from build123d import *

# Parameters (mm, degrees)
F0_R     = 7.14375
F0_R_2   = 33.3375
F0_R_3   = 8.509
F0_R_4   = 8.89
F0_R_5   = 137.31875
F1_DEPTH = 4.7625


with BuildPart() as f1:
    # F0 (on Right) → F1 (new body)
    with BuildSketch(Plane.YZ):
        with BuildLine():
            Line((-271.696104, -5.952033), (-271.696104, -221.890895))
            ThreePointArc((-271.696104, -221.890895), (-257.051472, -257.246163), (-221.696204, -271.890795))
            Line((-221.696204, -271.890795), (-6.535242, -271.890795))
            Line((-6.535242, -271.890795), (254.987282, -10.17713))
            ThreePointArc((254.987282, -10.17713), (250.021545, 250.150476), (-10.30357, 255.245143))
            Line((-10.30357, 255.245143), (-271.696104, -5.952033))
        make_face()
        with Locations((-244.518688, -244.572155)):
            Circle(F0_R, mode=Mode.SUBTRACT)
        with Locations((-34.20458, -244.572155)):
            Circle(F0_R, mode=Mode.SUBTRACT)
        with Locations((-244.518688, -34.39127)):
            Circle(F0_R, mode=Mode.SUBTRACT)
        with Locations((-190.572923, -34.39127)):
            Circle(F0_R, mode=Mode.SUBTRACT)
        with Locations((-127.660375, -34.39127)):
            Circle(F0_R_2, mode=Mode.SUBTRACT)
        with Locations((-64.7478, -34.39127)):
            Circle(F0_R, mode=Mode.SUBTRACT)
        with Locations((2.731567, 2.773934)):
            Circle(F0_R_3, mode=Mode.SUBTRACT)
        with Locations((81.847131, -140.540435)):
            Circle(F0_R, mode=Mode.SUBTRACT)
        with Locations((117.685388, -44.901637)):
            Circle(F0_R_3, mode=Mode.SUBTRACT)
        with Locations((231.706395, 2.789326)):
            Circle(F0_R_3, mode=Mode.SUBTRACT)
        with Locations((-140.560552, 81.726329)):
            Circle(F0_R, mode=Mode.SUBTRACT)
        with Locations((-44.795135, 117.578861)):
            Circle(F0_R_3, mode=Mode.SUBTRACT)
        with Locations((2.655392, 231.961842)):
            Circle(F0_R_4, mode=Mode.SUBTRACT)
        with Locations((117.211272, 117.405963)):
            Circle(F0_R_5, mode=Mode.SUBTRACT)
        with Locations((279.937693, 117.578861)):
            Circle(F0_R_3, mode=Mode.SUBTRACT)
        with Locations((117.600933, 279.905917)):
            Circle(F0_R_3, mode=Mode.SUBTRACT)
        with Locations((231.809138, 231.996234)):
            Circle(F0_R_3, mode=Mode.SUBTRACT)
    extrude(amount=F1_DEPTH)


solid = f1.part
Design review of the part built by this model. Coordinates are the model's own, in mm. Round coordinates to 2 decimals unless told otherwise and drop trailing zeros. Loops run counter-clockwise (first coordinate to the right, second up) from the corner with the lowest first, then second, coordinate; pieces in that order, holes last. Notation, with made-up numbers: (13, 54.5) - (20, 54.5) arc R32 cw to (20, 91.5) - close; hole circle Ø5 at (-25.5, 45). An arc over 180 degrees is marked (long way). One line per item, written item: value. Start each with the question number.
1) To check wall thickness, follow L1, parallel to Y at x = 2.65, z = -246.5; L2, parallel to Y at x = 3.25, z = 7; L3, parallel to Y at x = 1.95, z = 58. State the ranges of each line that lie inside material, in increasing order. Write a range as from..to.
2) Consider section C-C on x = 3.8. Give the number of separate pieces and of enclosed holes in the cut face, then the cut area to 3 significant figures.
3) Consider section B-B on y = 33.5. Give the boundary of the cut face in (x, z).
4) Consider section A-A on z = 145.5. Give the boundary of the cut face in (x, y), then the cut area to 3 significant figures.
5) Draft analysis for pull direction Z (two halves, no side actions). For faces 1 (the flat face through (2.348, 122.395, -142.866)), 2 (the cylindrical face through (2.348, 10.848, 5.33)), 3 (the cylindrical face through (2.348, 288.054, 120.135)), 4 (the cylindrical face through (2.35, 252.84, 247.27)), state which applies: +Z half, -Z half, draft (parallel to the pull), parting line (faces both ways), or undercut.
6) Consider section D-D on z = -185.5. Give the boundary of the cut face in (x, y), then the cut area to 3 significant figures.
7) Insertion check: pin 1 Ø19.5 at (y, z) = (231.71, 2.79) entering from +X; pin 2 Ø15.5 at (y, z) = (279.94, 117.58) entering from +X; pin 3 Ø2 at (x, y) = (2.5, 66) entering from -Z. Each pin has a flat end and moves straight along its axis. Give the tip position at first contact, or say it passes through.
Reported:
1. L1: y = -265.22..-251.4, -237.64..-41.08, -27.33..18.84
1. L2: y = -258.73..-4.65, 10.12..35.56, 198.86..224.31, 239.1..269.1
1. L3: y = -207.7..-6.59, 241.02..295.34
2. separate pieces: 1
2. enclosed holes: 17
2. area: 160,000 mm^2
3. outline: (0, -231.83) - (4.76, -231.83) - (4.76, 8.55) - (0, 8.55) - close; (0, 226.26) - (4.76, 226.26) - (4.76, 285.49) - (0, 285.49) - close
4. outline: (0, -120.13) - (4.76, -120.13) - (4.76, -17.2) - (0, -17.2) - close; (0, 251.63) - (4.76, 251.63) - (4.76, 302.87) - (0, 302.87) - close
4. area: 734 mm^2
5. face 1: -Z half
5. face 2: undercut
5. face 3: undercut
5. face 4: parting line
6. outline: (0, -271.7) - (4.76, -271.7) - (4.76, 79.79) - (0, 79.79) - close
6. area: 1,670 mm^2
7. pin 1: stops at x = 4.76
7. pin 2: passes through
7. pin 3: stops at z = -200.3
